```python
from build123d import *

# Parameters (mm, degrees)
F1_DEPTH  = 8.5
F3_DEPTH  = 68.6
F4_W      = 6
F4_H      = 2.45
F5_DEPTH  = 4.75
F6_R      = 2.225
F7_DEPTH  = 25
F8_R      = 1.2071067812
F9_R      = 1.207
F10_DEPTH = 3


with BuildPart() as f1:
    # F0 (on Top) → F1 (new body)
    with BuildSketch(Plane.XY):
        Polygon((0, 54), (0, 0), (83, 0), (83, 12), (3, 54), align=None)
    extrude(amount=F1_DEPTH)

    # F2 (on face) → F3 (cut)
    with BuildSketch(Plane.XZ):
        Polygon((9.015292082, 4.25), (4.265292082, 4.25), (4.265292082, 2.8787931107), (6.640292082, 1.5075862213), (9.015292082, 2.8787931107), align=None)
        Polygon((4.265292082, 5.6212068893), (4.265292082, 4.25), (9.015292082, 4.25), (9.015292082, 5.6212068893), (6.640292082, 6.9924137787), align=None)
        Polygon((18.96107, 5.6789419162), (18.96107, 4.25), (21.43607, 4.25), (23.91107, 4.25), (23.91107, 5.6789419162), (21.43607, 7.1078838325), align=None)
        Polygon((21.43607, 4.25), (18.96107, 4.25), (18.96107, 2.8210580838), (21.43607, 1.3921161675), (23.91107, 2.8210580838), (23.91107, 4.25), align=None)
        Polygon((33.95607, 5.1044783984), (33.95607, 4.25), (35.43607, 4.25), (36.91607, 4.25), (36.91607, 5.1044783984), (35.43607, 5.9589567968), align=None)
        Polygon((35.43607, 4.25), (33.95607, 4.25), (33.95607, 3.3955216016), (35.43607, 2.5410432032), (36.91607, 3.3955216016), (36.91607, 4.25), align=None)
        with BuildLine():
            Line((49.43607, 4.25), (47.92107, 4.25))
            ThreePointArc((47.92107, 4.25), (49.43607, 2.735), (50.95107, 4.25))
            Line((50.95107, 4.25), (49.43607, 4.25))
        make_face()
        with BuildLine():
            ThreePointArc((50.95107, 4.25), (49.43607, 5.765), (47.92107, 4.25))
            Line((47.92107, 4.25), (49.43607, 4.25))
            Line((49.43607, 4.25), (50.95107, 4.25))
        make_face()
        Polygon((62.20107, 4.9630275824), (62.20107, 4.25), (63.43607, 4.25), (64.67107, 4.25), (64.67107, 4.9630275824), (63.43607, 5.6760551649), align=None)
        Polygon((63.43607, 4.25), (62.20107, 4.25), (62.20107, 3.5369724176), (63.43607, 2.8239448351), (64.67107, 3.5369724176), (64.67107, 4.25), align=None)
        Polygon((77.43607, 4.25), (76.45607, 4.25), (76.45607, 3.6841967362), (77.43607, 3.1183934724), (78.41607, 3.6841967362), (78.41607, 4.25), align=None)
        Polygon((76.45607, 4.8158032638), (76.45607, 4.25), (77.43607, 4.25), (78.41607, 4.25), (78.41607, 4.8158032638), (77.43607, 5.3816065276), align=None)
    extrude(amount=-F3_DEPTH, mode=Mode.SUBTRACT)

    # F4 (on face) → F5 (join)
    with BuildSketch(Plane.XY.offset(8.5)):
        with Locations((30.2142857143, 17.5765829772)):
            Rectangle(F4_W, F4_H)
        with Locations((24.2142857143, 20.0265829772)):
            Rectangle(F4_W, F4_H)
        with Locations((24.2142857143, 17.5765829772)):
            Rectangle(F4_W, F4_H)
        with Locations((30.2142857143, 20.0265829772)):
            Rectangle(F4_W, F4_H)
    extrude(amount=F5_DEPTH)

    # F6 (on face) → F7 (cut)
    with BuildSketch(Plane.YZ.offset(33.2142857143)):
        with Locations((18.8015829772, 10.875)):
            Circle(F6_R)
    extrude(amount=-F7_DEPTH, mode=Mode.SUBTRACT)

    # F8
    f8_edges = [f1.edges().sort_by_distance(p)[0] for p in [
        (27.214286, 21.251583, 13.25),
    ]]
    fillet(f8_edges, radius=F8_R)

    # F9
    f9_edges = [f1.edges().sort_by_distance(p)[0] for p in [
        (27.214286, 16.351583, 13.25),
    ]]
    fillet(f9_edges, radius=F9_R)

    # F10 (cut): a face of the model
    f10_faces = [f1.faces().sort_by_distance(p)[0] for p in [
        (27.2142857143, 18.8015295866, 13.25),
    ]]
    extrude(f10_faces, amount=-F10_DEPTH, mode=Mode.SUBTRACT)


solid = f1.part
```
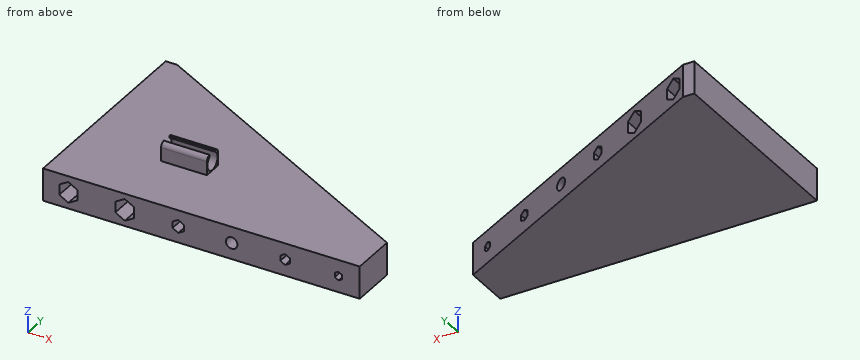
Geometry check sheet. Reference: the model listing, model coordinates, mm. Coordinates: 2 decimals unless noted, no trailing zeros. Write each loop counter-clockwise with the first axis right and the second up, starting at its lowest first coordinate (ties: lowest second). Pieces come first, ordered by that corner, then holes. Notation, with made-up numbers: (22.25, -36.5) -> (63.25, -36.5) arc R19 ccw to (63.25, -8.5) -> close; hole circle Ø8 at (-2, 9.25). An arc over 180 degrees is marked (long way). Use CSV: the item, a comma, the result in double quotes. Start each with the question number.
Item 1: Cross-section at D-D, the plane x = 70.5. Record the cut outline in (y, z), plus the area to 3 significant figures.
Item 2: Thickness scan on line 1 (X direction, y = 31, z = 6.5); line 2 (Z direction, x = 65.5, y = 15.5); line 3 (Y direction, x = 31, z = 10.25). Record the ranges inside material, lowest first.
Item 3: Depth check by flat-ended pin: pin 1 Ø2 at (y, z) = (47, 9) entering from +X; pin 2 Ø0.9 at (y, z) = (25, 4.5) entering from +X; pin 3 Ø4 at (y, z) = (18.5, 12) entering from +X; pin 4 Ø2.5 at (x, z) = (49.44, 4.25) entering from +Y. Enter the tip coordinate at first touch or a pass-through.
Item 4: Cross-section at C-C, the plane x = 40. Record the cut outline in (y, z) (3 decimals), plus the area to 3 significant figures.
Item 5: Cross-section at B-B, the plane y = 40. Record the cut outline in (x, z).
Answers:
1,outline,"(0, 0) -> (18.56, 0) -> (18.56, 8.5) -> (0, 8.5) -> close"
1,area,"158 mm^2"
2,line 1,"0 to 5.79, 7.49 to 20.38, 22.49 to 46.81"
2,line 2,"0 to 8.5"
2,line 3,"16.35 to 16.67, 20.94 to 21.25"
3,pin 1,"x = 17.98"
3,pin 2,"x = 59.1"
3,pin 3,"x = 33.21"
3,pin 4,"through"
4,outline,"(0, 0) -> (34.575, 0) -> (34.575, 8.5) -> (0, 8.5) -> close"
4,area,"294 mm^2"
5,outline,"(0, 0) -> (29.67, 0) -> (29.67, 8.5) -> (0, 8.5) -> close; hole (4.27, 2.88) -> (6.64, 1.51) -> (9.02, 2.88) -> (9.02, 5.62) -> (6.64, 6.99) -> (4.27, 5.62) -> close; hole (18.96, 2.82) -> (21.44, 1.39) -> (23.91, 2.82) -> (23.91, 5.68) -> (21.44, 7.11) -> (18.96, 5.68) -> close"
